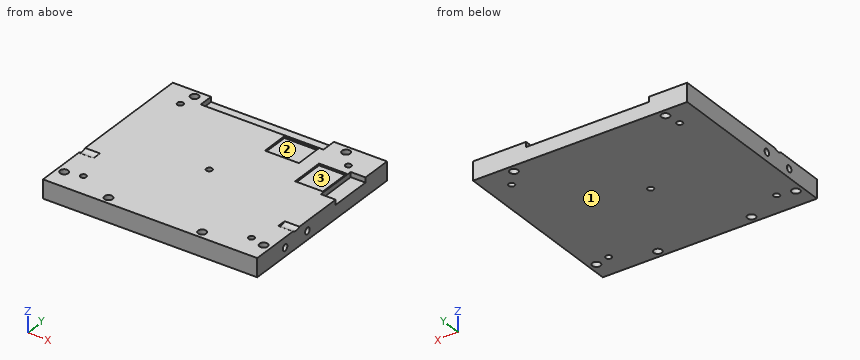
```python
from build123d import *

# Parameters (mm, degrees)
MAIN_STOCK_START                 = -2.751909566
SKETCH_1_W                       = 57.95
SKETCH_1_H                       = 49.98
MAIN_STOCK_DEPTH                 = 5
SKETCH_2_R                       = 1.1
FRAME_6XD2P2_THROUGH_DEPTH       = 71.63982517
SKETCH_3_R                       = 0.8
PCB_5XD1P6_M2_THROUGH_DEPTH      = 71.63982517
SKETCH_4_R                       = 2.05
SMA_L_CENTER_MATCHING_ARC_DEPTH  = 4
SKETCH_5_R                       = 0.875
SMA_L_LOWER_2XD1P75_BLIND4_DEPTH = 4
SMA_R_CENTER_MATCHING_ARC_START  = -4
SKETCH_6_R                       = 2.05
SMA_R_CENTER_MATCHING_ARC_DEPTH  = 4
SMA_R_LOWER_2XD1P75_BLIND4_START = -4
SKETCH_7_R                       = 0.875
SMA_R_LOWER_2XD1P75_BLIND4_DEPTH = 4
SKETCH_8_W                       = 6.7
SKETCH_8_H                       = 11.5
RIGHT_TYPEC_WINDOW_LOWER_DEPTH   = 4
SKETCH_9_W                       = 33.203
SKETCH_9_H                       = 6.7
REAR_WINDOW_LOWER_DEPTH          = 4
SKETCH_10_W                      = 7.5
SKETCH_10_H                      = 9.2
TYPEC_BOTTOM_RECESS_A_DEPTH      = 0.5
SKETCH_11_W                      = 9.2
SKETCH_11_H                      = 7.5
TYPEC_BOTTOM_RECESS_B_DEPTH      = 0.5


with BuildPart() as part:
    # 草图1 → Main_Stock (new body)
    with BuildSketch(Plane.XY.offset(MAIN_STOCK_START)):
        with Locations((24.675, 20.69)):
            Rectangle(SKETCH_1_W, SKETCH_1_H)
    extrude(amount=MAIN_STOCK_DEPTH)

    # 草图2 → Frame_6xD2p2_Through (cut, through all)
    with BuildSketch(Plane.XY.offset(2.248090434)):
        with Locations((-2.3, 1)):
            Circle(SKETCH_2_R)
        with Locations((51.65, 1)):
            Circle(SKETCH_2_R)
        with Locations((12, -2.3)):
            Circle(SKETCH_2_R)
        with Locations((37.35, -2.3)):
            Circle(SKETCH_2_R)
        with Locations((3, 43.68)):
            Circle(SKETCH_2_R)
        with Locations((44, 43.68)):
            Circle(SKETCH_2_R)
    extrude(amount=-FRAME_6XD2P2_THROUGH_DEPTH, mode=Mode.SUBTRACT)

    # 草图3 → PCB_5xD1p6_M2_Through (cut, through all)
    with BuildSketch(Plane.XY.offset(2.248090434)):
        with Locations((23.428293927, 20.276755792)):
            Circle(SKETCH_3_R)
        with Locations((2.206251763, 39.333791606)):
            Circle(SKETCH_3_R)
        with Locations((47.653340917, 39.333791606)):
            Circle(SKETCH_3_R)
        with Locations((47.653340917, 1.976720232)):
            Circle(SKETCH_3_R)
        with Locations((2.206251763, 1.976720232)):
            Circle(SKETCH_3_R)
    extrude(amount=-PCB_5XD1P6_M2_THROUGH_DEPTH, mode=Mode.SUBTRACT)

    # 草图4 → SMA_L_Center_Matching_Arc (cut)
    with BuildSketch(Plane.ZY.offset(4.3)):
        with Locations((3.899496327, 10.725)):
            Circle(SKETCH_4_R)
    extrude(amount=-SMA_L_CENTER_MATCHING_ARC_DEPTH, mode=Mode.SUBTRACT)

    # 草图5 → SMA_L_Lower_2xD1p75_Blind4 (cut)
    with BuildSketch(Plane.ZY.offset(4.3)):
        with Locations((-0.400503673, 6.425)):
            Circle(SKETCH_5_R)
        with Locations((-0.400503673, 15.025)):
            Circle(SKETCH_5_R)
    extrude(amount=-SMA_L_LOWER_2XD1P75_BLIND4_DEPTH, mode=Mode.SUBTRACT)

    # 草图6 → SMA_R_Center_Matching_Arc (cut)
    with BuildSketch(Plane(origin=(53.65, 0, 0), x_dir=(0, 0, -1), z_dir=(1, 0, 0)).offset(SMA_R_CENTER_MATCHING_ARC_START)):
        with Locations((-3.899496327, 10.725)):
            Circle(SKETCH_6_R)
    extrude(amount=SMA_R_CENTER_MATCHING_ARC_DEPTH, mode=Mode.SUBTRACT)

    # 草图7 → SMA_R_Lower_2xD1p75_Blind4 (cut)
    with BuildSketch(Plane(origin=(53.65, 0, 0), x_dir=(0, 0, -1), z_dir=(1, 0, 0)).offset(SMA_R_LOWER_2XD1P75_BLIND4_START)):
        with Locations(Location((0.400503673, 6.425, 0), (0, 0, 180))):
            Circle(SKETCH_7_R)
        with Locations(Location((0.400503673, 15.025, 0), (0, 0, 180))):
            Circle(SKETCH_7_R)
    extrude(amount=SMA_R_LOWER_2XD1P75_BLIND4_DEPTH, mode=Mode.SUBTRACT)

    # 草图8 → Right_TypeC_Window_Lower (cut)
    with BuildSketch(Plane(origin=(53.65, 0, 0), x_dir=(0, 0, -1), z_dir=(1, 0, 0))):
        with Locations((-4.25, 31.65)):
            Rectangle(SKETCH_8_W, SKETCH_8_H)
    extrude(amount=-RIGHT_TYPEC_WINDOW_LOWER_DEPTH, mode=Mode.SUBTRACT)

    # 草图9 → Rear_Window_Lower (cut)
    with BuildSketch(Plane(origin=(0, 45.68, 0), x_dir=(1, 0, 0), z_dir=(0, 1, 0))):
        with Locations((22.6715, -4.25)):
            Rectangle(SKETCH_9_W, SKETCH_9_H)
    extrude(amount=-REAR_WINDOW_LOWER_DEPTH, mode=Mode.SUBTRACT)

    # 草图10 → TypeC_Bottom_Recess_A (cut)
    with BuildSketch(Plane.XY.offset(2.248090434)):
        with Locations((45.6, 31.7)):
            Rectangle(SKETCH_10_W, SKETCH_10_H)
    extrude(amount=-TYPEC_BOTTOM_RECESS_A_DEPTH, mode=Mode.SUBTRACT)

    # 草图11 → TypeC_Bottom_Recess_B (cut)
    with BuildSketch(Plane.XY.offset(2.248090434)):
        with Locations((33.523, 37.63)):
            Rectangle(SKETCH_11_W, SKETCH_11_H)
    extrude(amount=-TYPEC_BOTTOM_RECESS_B_DEPTH, mode=Mode.SUBTRACT)


solid = part.part
```
CAD build for the part. Positions are in the model's coordinates, mm. Face numbers are marked on the shaded views. Round coordinates to 2 decimals unless told otherwise and drop trailing zeros. Order: outer loops, then holes, each group sorted by start corner. A loop starts at its lowest first (then second) coordinate and runs counter-clockwise, first axis right, second up. Notation, with made-up numbers: (0, 17.5) -> (44, 17.5) arc R6 ccw to (44, 21.5) -> close; hole circle Ø1 at (-10, 63). An arc over 180 degrees is marked (long way). One line per question, with ' | ' between items.
Q1. Slice it at B-B (x = 44). Write the cut outline in (y, z).
Completed:
outline: (-4.3, -2.75) -> (42.58, -2.75) -> (42.58, 2.25) -> (36.3, 2.25) -> (36.3, 1.75) -> (27.1, 1.75) -> (27.1, 2.25) -> (-4.3, 2.25) -> close; (44.78, -2.75) -> (45.68, -2.75) -> (45.68, 2.25) -> (44.78, 2.25) -> close
Q2. Drop flat-ended pins along their axis: pin 1 (2 mm diameter, centred on x = 51.5, y = 34, fed in from +Z); pin 2 (0.5 mm diameter, centred on y = 6.5, z = -0.5, fed in from -X). Give the stop position or say it passes through.
Completed:
pin 1: stops at z = 0.9 | pin 2: stops at x = -0.3
Q3. Probe probe 1 along X at (y, z) = (34.5, 2); probe 2 along Y at (x, z) = (51.65, -0.35); probe 3 along Y at (x, z) = (44, -1.4). List the from-to ranges inside material, lowest first.
Completed:
probe 1: x = -4.3 to 28.92, 38.12 to 41.85, 49.35 to 49.65 | probe 2: y = -4.3 to -0.1, 2.1 to 5.55, 7.3 to 14.15, 15.9 to 45.68 | probe 3: y = -4.3 to 42.58, 44.78 to 45.68
Q4. Slice it at D-D (x = 30). Write the cut outline in (y, z), then the cut area to 3 significant figures.
Completed:
outline: (-4.3, -2.75) -> (45.68, -2.75) -> (45.68, 0.9) -> (41.68, 0.9) -> (41.68, 2.25) -> (41.38, 2.25) -> (41.38, 1.75) -> (33.88, 1.75) -> (33.88, 2.25) -> (-4.3, 2.25) -> close | area: 241 mm^2
Q5. Slice it at C-C (x = 51.65). Give the number of separate pieces and of enclosed holes in the cut face, then the cut area to 3 significant figures.
Completed:
separate pieces: 2 | enclosed holes: 2 | area: 218 mm^2
Q6. Two-plate mould, pull along X, no slides. Class the marked faces 1, 2 and 3: released by +X, released by -X, zero draft, split by the parting line, or undercut.
Completed:
face 1: zero draft | face 2: undercut | face 3: undercut
Q7. Slice it at A-A (y = 43.68). Write the cut outline in (x, z).
Completed:
outline: (-4.3, -2.75) -> (1.9, -2.75) -> (1.9, 2.25) -> (-4.3, 2.25) -> close; (4.1, -2.75) -> (42.9, -2.75) -> (42.9, 2.25) -> (39.27, 2.25) -> (39.27, 0.9) -> (6.07, 0.9) -> (6.07, 2.25) -> (4.1, 2.25) -> close; (45.1, -2.75) -> (53.65, -2.75) -> (53.65, 2.25) -> (45.1, 2.25) -> close
